The model under review builds one solid part; all positions refer to its coordinate system, in mm. Face numbers are marked on the shaded views. A direction names the side the tool comes from. Coordinates: 2 decimals unless noted, no trailing zeros. Loops run counter-clockwise (first coordinate to the right, second up) from the corner with the lowest first, then second, coordinate; pieces in that order, holes last. Notation, with made-up numbers: (26.5, 60) - (35.5, 60) arc R27 ccw to (35.5, 79) - close; hole circle Ø1 at (21.5, -38.5). An arc over 180 degrees is marked (long way). One line per item, written item: value. Start each with the question number.
1. We need section D-D, the plane x = -2.3. Give the boundary of the cut face in (y, z), then the cut area to 3 significant figures.
2. We need section A-A, the plane z = 0. Count the separate pieces of the cut face and the enclosed holes in it, then the cut area to 3 significant figures.
3. Insertion check: P1, Ø3, axis at y = -8, z = 0, coming from the -X side; P2, Ø1.2, axis at y = -5.66, z = -5.66, coming from the -X side (3 decimals); P3, Ø1.8, axis at y = 1, z = 0, coming from the +X side; P4, Ø2, axis at x = 0.5, y = 8, coming from the +Z side. Each pin has a flat end and moves straight along its axis. Give the tip position at first contact, or say it passes through.
4. Mouldability with a two-part tool opening along Z and no side actions: class the marked faces 4, 5 and 6 as +Z half, -Z half, draft (parallel to the pull), parting line (faces both ways), or undercut.
5. For the marked faces 1, 2 and 3, list the 3-axis set-ups (+Z, -Z, +X, -X, +Y, -Y) from which the entire face can be reached by the end or side of a thin tool; tool diameter is ignored.
6. To check wall thickness, follow line 1 (Y direction, x = -0.2, z = 0); line 2 (Z direction, x = -0.2, y = -5.75); line 3 (Z direction, x = 0.4, y = -5). State the ranges of each line that lie inside material, in increasing order.
from build123d import *

# Parameters (mm, degrees)
SKETCH2_R          = 1
CUT_EXTRUDE1_DEPTH = 16.842979518
CIRPATTERN1_COUNT  = 8
CHAMFER1_SIZE      = 0.2


with BuildPart() as part:
    # Sketch1 → Revolve1 (revolve)
    with BuildSketch(Plane.XY, mode=Mode.PRIVATE) as revolve1_sk:
        Polygon((1, 11), (-1, 11), (-1, 3.75), (-4, 3.75), (-4, 1.5), (-3.5, 1.5), (-3.5, 3), (1, 3), align=None)
    revolve(revolve1_sk.sketch.rotate(Axis((0, 0, 0), (1, 0, 0)), 90), axis=Axis((0, 0, 0), (1, 0, 0)))

    # Sketch2 → Cut-Extrude1 (cut, through all)
    with BuildSketch(Plane.ZY.offset(1)):
        with Locations((0, 8)):
            Circle(SKETCH2_R)
    cut_extrude1 = extrude(amount=-CUT_EXTRUDE1_DEPTH, mode=Mode.SUBTRACT)

    # CirPattern1: Cut-Extrude1 ×8 about axis
    cirpattern1_axis = Axis((0, 0, 0), (1, 0, 0))
    for i in range(1, CIRPATTERN1_COUNT):
        add(cut_extrude1.rotate(cirpattern1_axis, i * 360 / CIRPATTERN1_COUNT), mode=Mode.SUBTRACT)

    # Chamfer1
    chamfer1_edges = [part.edges().sort_by_distance(p)[0] for p in [
        (-1, 8, -1),
        (-1, 4.949747468, -6.363961031),
        (-1, -1, -8),
        (-1, -6.363961031, -4.949747468),
        (-1, -8, 1),
        (-1, -4.949747468, 6.363961031),
        (-1, 1, 8),
        (-1, 6.363961031, 4.949747468),
        (-4, 0, -3.75),
        (-1, 0, -11),
    ]]
    chamfer(chamfer1_edges, length=CHAMFER1_SIZE)


solid = part.part
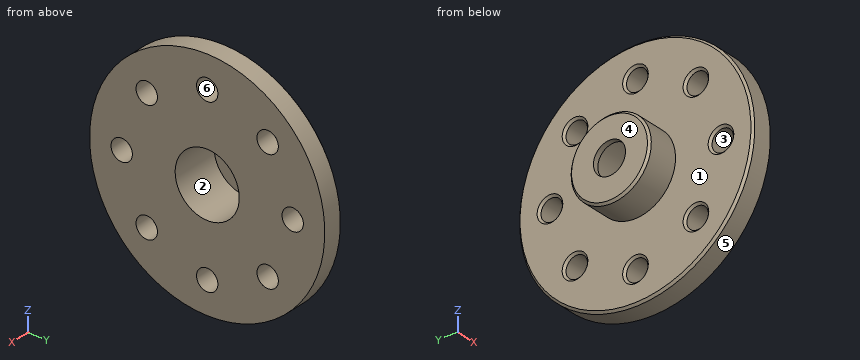
Findings below:
1. outline: circle Ø7.5 at (0, 0); hole circle Ø6 at (0, 0)
1. area: 15.9 mm2
2. separate pieces: 4
2. enclosed holes: 0
2. area: 29.8 mm2
3. P1: x = -1
3. P2: through
3. P3: x = -3.5
3. P4: z = 8.49
4. face 4: draft
4. face 5: parting line
4. face 6: undercut
5. face 1: -X
5. face 2: +X
5. face 3: +X, -X
6. line 1: -11 to -9, -7 to -3, 3 to 7, 9 to 11
6. line 2: -9.38 to -6.65, -4.66 to 4.66, 6.65 to 9.38
6. line 3: -9.8 to -6.41, -4.9 to 4.9, 6.41 to 9.8
